Verification items for the finished model (mm, model axes). Face numbers are marked on the shaded views. A direction names the side the tool comes from. Coordinates: 2 decimals unless noted, no trailing zeros. Loops run counter-clockwise (first coordinate to the right, second up) from the corner with the lowest first, then second, coordinate; pieces in that order, holes last.
Q1. Material ranges on probe 1 along Z at (x, y) = (8, 2.2); probe 2 along X at (y, z) = (3.35, -5); probe 3 along Z at (x, y) = (5, 0.7), recorded low to high.
Q2. Mould release check, pull along Z, two halves, no side actions. Record for the marked faces 3, 4, 5 and 6: +Z half, -Z half, draft (parallel to the pull), parting line (faces both ways), or undercut.
Q3. Sectioned sample at B-B (y = 3.15). Enter the section's corners in (x, z).
Q4. Sectioned sample at A-A (x = 5). Enter the section's corners in (y, z), then the cut area to 3 significant figures.
Q5. Go/stop test with a flat-tipped pin: P1, Ø1.3, axis at x = 10, z = -5, coming from the -Y side. Record where the tip stops, or that it passes through.
Q6. Sectioned sample at C-C (z = -4.5). Enter the section's corners in (x, y).
Q7. Access from +Z, -Z, +X, -X, +Y, -Y to the whole of each face (thin tool, end or side, straight path). Record for the marked faces 1 and 2.
Q8. Sectioned sample at D-D (z = -8.6). Enter the section's corners in (x, y).
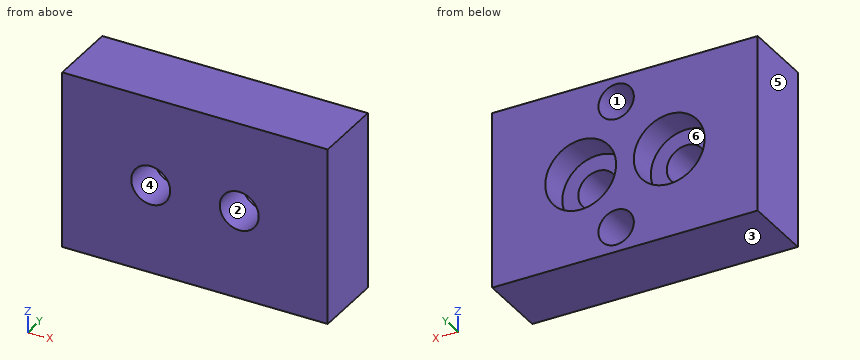
```python
from build123d import *

# Parameters (mm, degrees)
SKETCH_1_W          = 15
SKETCH_1_H          = 10
EXTRUDE_1_DEPTH     = 4
SKETCH_2_R          = 1.1
CUT_EXTRUDE_1_DEPTH = 5
SKETCH_5_R          = 1
CUT_EXTRUDE_4_DEPTH = 3
SKETCH_3_R          = 2
CUT_EXTRUDE_5_DEPTH = 1.7


with BuildPart() as part:
    # 草图1 → 凸台-拉伸1 (new body)
    with BuildSketch(Plane(origin=(0, 0, 0), x_dir=(1, 0, 0), z_dir=(0, 1, 0))):
        with Locations((7.5, 5)):
            Rectangle(SKETCH_1_W, SKETCH_1_H)
    extrude(amount=EXTRUDE_1_DEPTH)

    # 草图2 → 切除-拉伸1 (cut, through all)
    with BuildSketch(Plane(origin=(0, 4, 0), x_dir=(1, 0, 0), z_dir=(0, 1, 0))):
        with Locations((5, 5)):
            Circle(SKETCH_2_R)
        with Locations((10, 5)):
            Circle(SKETCH_2_R)
    extrude(amount=-CUT_EXTRUDE_1_DEPTH, mode=Mode.SUBTRACT)

    # 草图5 → 切除-拉伸4 (cut)
    with BuildSketch(Plane(origin=(0, 4, 0), x_dir=(1, 0, 0), z_dir=(0, 1, 0))):
        with Locations((8, 8.6)):
            Circle(SKETCH_5_R)
        with Locations((8, 1.4)):
            Circle(SKETCH_5_R)
    extrude(amount=-CUT_EXTRUDE_4_DEPTH, mode=Mode.SUBTRACT)

    # 草图3 → 切除-拉伸5 (cut)
    with BuildSketch(Plane(origin=(0, 4, 0), x_dir=(1, 0, 0), z_dir=(0, 1, 0))):
        with Locations((5, 5)):
            Circle(SKETCH_3_R)
        with Locations((10, 5)):
            Circle(SKETCH_3_R)
    extrude(amount=-CUT_EXTRUDE_5_DEPTH, mode=Mode.SUBTRACT)


solid = part.part
```
Geometry check:
1. probe 1: z = -10 to -9.6, -7.6 to -2.4, -0.4 to 0
1. probe 2: x = 0 to 3, 7 to 8, 12 to 15
1. probe 3: z = -10 to -6.1, -3.9 to 0
2. face 3: -Z half
2. face 4: undercut
2. face 5: draft
2. face 6: undercut
3. outline: (0, -10) - (15, -10) - (15, 0) - (0, 0) - close; hole circle Ø4 at (5, -5); hole circle Ø2 at (8, -8.6); hole circle Ø2 at (8, -1.4); hole circle Ø4 at (10, -5)
4. outline: (0, -10) - (4, -10) - (4, -7) - (2.3, -7) - (2.3, -6.1) - (0, -6.1) - close; (0, -3.9) - (2.3, -3.9) - (2.3, -3) - (4, -3) - (4, 0) - (0, 0) - close
4. area: 28.1 mm2
5. P1: passes through
6. outline: (0, 0) - (4.02, 0) - (4.02, 2.3) - (3.06, 2.3) - (3.06, 4) - (0, 4) - close; (5.98, 0) - (9.02, 0) - (9.02, 2.3) - (8.06, 2.3) - (8.06, 4) - (6.94, 4) - (6.94, 2.3) - (5.98, 2.3) - close; (10.98, 0) - (15, 0) - (15, 4) - (11.94, 4) - (11.94, 2.3) - (10.98, 2.3) - close
7. face 1: +Y
7. face 2: +Y, -Y
8. outline: (0, 0) - (15, 0) - (15, 4) - (9, 4) - (9, 1) - (7, 1) - (7, 4) - (0, 4) - close
